CAD build for the part. Positions are in the model's coordinates, mm. Round coordinates to 2 decimals unless told otherwise and drop trailing zeros. Order: outer loops, then holes, each group sorted by start corner. A loop starts at its lowest first (then second) coordinate and runs counter-clockwise, first axis right, second up. Notation, with made-up numbers: (57.5, 31.25) -> (100.5, 31.25) arc R35 cw to (100.5, 67.25) -> close; hole circle Ø8 at (-15, 63). An arc over 180 degrees is marked (long way). Return JSON: item names as keys, results as strings. Group by question number.
Q1. Probe line 1 along Y through (x, z) = (108, 1.75); line 2 along Y through (x, z) = (123, 0.65); line 3 along Y through (x, z) = (121, 2.2). List the from-to ranges inside material, lowest first.
Q2. Cut at D-D (x = 121.5). Write the cut outline in (y, z) (3 decimals).
Q3. Cut at B-B (y = 113.5). Write the cut outline in (x, z) (3 decimals).
Q4. Flat gauge pin, fed straight in: pin 1 (6 mm diameter, centred on x = 91.75, y = 147.1, fed in from +Z) (3 decimals). Where does the tip first touch, or does it go through?
Q5. Cut at A-A (x = 114). Write the cut outline in (y, z) (3 decimals), then the cut area to 3 significant figures.
Q6. Cut at C-C (z = 1.55). Count the separate pieces of the cut face and the enclosed holes in it, then the cut area to 3 significant figures.
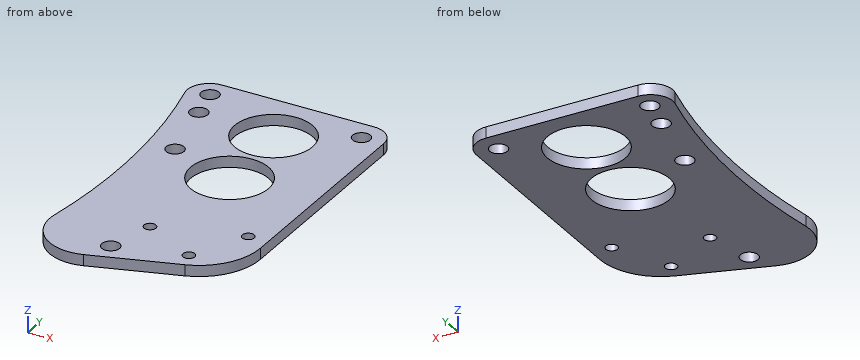
from build123d import *

# Parameters (mm, degrees)
SKETCH2_R           = 2.5527
SKETCH2_R_2         = 11.176
SKETCH2_R_3         = 1.7
BOSS_EXTRUDE1_DEPTH = 3.175


with BuildPart() as part:
    # Sketch2 → Boss-Extrude1 (new body)
    with BuildSketch(Plane.XY):
        with BuildLine():
            Line((89.804840449, 162.158224077), (133.35, 162.158224077))
            ThreePointArc((133.35, 162.158224077), (137.840128061, 160.298352138), (139.7, 155.808224077))
            Line((139.7, 155.808224077), (139.7, 93.800599977))
            ThreePointArc((139.7, 93.800599977), (136.352183067, 83.506635024), (127.589632634, 77.151219806))
            Line((127.589632634, 77.151219806), (103.12742621, 69.232468195))
            ThreePointArc((103.12742621, 69.232468195), (90.956620775, 71.66782369), (86.675019958, 83.318032089))
            ThreePointArc((86.675019958, 83.318032089), (88.737860448, 118.949701892), (83.642604572, 154.275465457))
            ThreePointArc((83.642604572, 154.275465457), (84.802065357, 159.719073266), (89.804840449, 162.158224077))
        make_face()
        with Locations((89.657841737, 156.395094021)):
            Circle(SKETCH2_R, mode=Mode.SUBTRACT)
        with Locations((91.747700228, 147.102187237)):
            Circle(SKETCH2_R, mode=Mode.SUBTRACT)
        with Locations((106.775437357, 76.433708644)):
            Circle(SKETCH2_R, mode=Mode.SUBTRACT)
        with Locations((115.1001, 121.545060726)):
            Circle(SKETCH2_R_2, mode=Mode.SUBTRACT)
        with Locations((113.962375762, 145.648224077)):
            Circle(SKETCH2_R_2, mode=Mode.SUBTRACT)
        with Locations((133.35, 155.808224077)):
            Circle(SKETCH2_R, mode=Mode.SUBTRACT)
        with Locations((95.988414932, 127.701170501)):
            Circle(SKETCH2_R, mode=Mode.SUBTRACT)
        with Locations((134.09377421, 97.646134406)):
            Circle(SKETCH2_R_3, mode=Mode.SUBTRACT)
        with Locations((126.045534429, 81.906825767)):
            Circle(SKETCH2_R_3, mode=Mode.SUBTRACT)
        with Locations((110.30622579, 89.955065547)):
            Circle(SKETCH2_R_3, mode=Mode.SUBTRACT)
    extrude(amount=BOSS_EXTRUDE1_DEPTH)


solid = part.part
Solution:
{
 "1": {"line 1": "y = 70.81 to 74.19, 78.67 to 112.91, 130.18 to 136.2, 155.1 to 162.16", "line 2": "y = 75.67 to 113.64, 129.45 to 139.07, 152.22 to 162.16", "line 3": "y = 75.02 to 112.05, 131.04 to 136.97, 154.33 to 162.16"},
 "2": {"outline": "(75.18, 0) -> (112.383, 0) -> (112.383, 3.175) -> (75.18, 3.175) -> close; (130.707, 0) -> (137.397, 0) -> (137.397, 3.175) -> (130.707, 3.175) -> close; (153.9, 0) -> (162.158, 0) -> (162.158, 3.175) -> (153.9, 3.175) -> close"},
 "3": {"outline": "(88.887, 0) -> (107.343, 0) -> (107.343, 3.175) -> (88.887, 3.175) -> close; (122.858, 0) -> (139.7, 0) -> (139.7, 3.175) -> (122.858, 3.175) -> close"},
 "4": {"pin 1": "stops at z = 3.175"},
 "5": {"outline": "(72.752, 0) -> (110.423, 0) -> (110.423, 3.175) -> (72.752, 3.175) -> close; (132.667, 0) -> (134.472, 0) -> (134.472, 3.175) -> (132.667, 3.175) -> close; (156.824, 0) -> (162.158, 0) -> (162.158, 3.175) -> (156.824, 3.175) -> close", "area": "142 mm²"},
 "6": {"separate pieces": "1", "enclosed holes": "10", "area": "3,690 mm²"}
}
